Part model, mm, in its own coordinate system. Round coordinates to 2 decimals unless told otherwise and drop trailing zeros. Write each loop counter-clockwise with the first axis right and the second up, starting at its lowest first coordinate (ties: lowest second). Pieces come first, ordered by that corner, then holes. Notation, with made-up numbers: (82.25, 5) -> (96.25, 5) arc R9 ccw to (96.25, 11) -> close; hole circle Ø3 at (19, 7). An arc over 180 degrees is marked (long way). Return JSON: item names as keys, results as strings. Group by question number.
(1) Saw through at A-A (z = 0). List the corners of the cut face in (x, y).
(2) Saw through at B-B (y = -498.5). List the corners of the cut face in (x, z), plus the area to 3 significant figures.
(3) Drill centre lines: L1, parallel to X at y = 0, z = 564.5; L2, parallel to Z at x = 8, y = 279; L3, parallel to Y at x = -3, z = 473.5. Where is each one in solid material? Low to high. Write a range as from..to.
(4) Drop flat-ended pins along their axis: pin 1 Ø1 at (x, y) = (3.5, 126) entering from -Z; pin 2 Ø12 at (x, y) = (-4, -348) entering from +Z; pin 3 Ø3 at (x, y) = (4.5, 319) entering from -Z. Give the stop position or say it passes through.
from build123d import *

# Parameters (mm, degrees)
SKETCH012_R      = 5
EXTRUDE012_DEPTH = 1500
SKETCH001_R      = 570
SKETCH001_R_2    = 550
EXTRUDE_DEPTH    = 10


with BuildPart() as extrude012:
    # Sketch012 (on Face1 of Extrude011) → Extrude012 (new body)
    with BuildSketch(Plane.XY.offset(650)):
        Circle(SKETCH012_R)
    extrude(amount=-EXTRUDE012_DEPTH)


with BuildPart() as cut:
    # Sketch001 → Extrude (new body, symmetric)
    with BuildSketch(Plane.YZ):
        Circle(SKETCH001_R)
        Circle(SKETCH001_R_2, mode=Mode.SUBTRACT)
    extrude(amount=EXTRUDE_DEPTH, both=True)

    # Cut: cut Extrude012
    add(extrude012.part, mode=Mode.SUBTRACT)


solid = cut.part
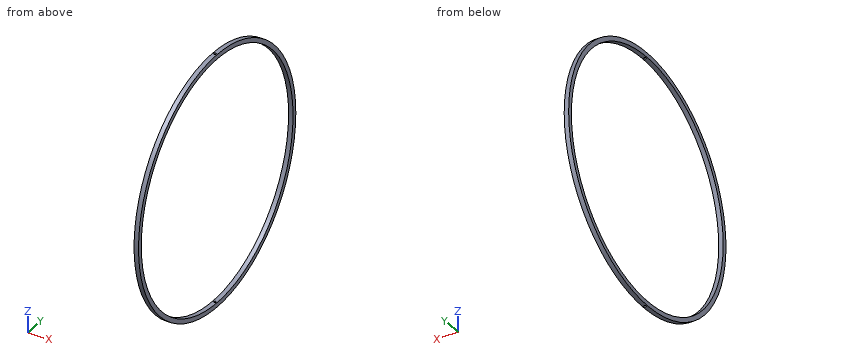
Computed values:
{
 "1": {"outline": "(-10, -570) -> (10, -570) -> (10, -550) -> (-10, -550) -> close; (-10, 550) -> (10, 550) -> (10, 570) -> (-10, 570) -> close"},
 "2": {"outline": "(-10, -276.4) -> (10, -276.4) -> (10, -232.37) -> (-10, -232.37) -> close; (-10, 232.37) -> (10, 232.37) -> (10, 276.4) -> (-10, 276.4) -> close", "area": "1,760 mm2"},
 "3": {"L1": "-10..-5, 5..10", "L2": "-497.05..-473.98, 473.98..497.05", "L3": "-317.33..-279.82, 279.82..317.33"},
 "4": {"pin 1": "z = -556.01", "pin 2": "z = 456", "pin 3": "z = -473.39"}
}
